from build123d import *

# Parameters (mm, degrees)
BOSS_EXTRUDE1_DEPTH = 6
FILLET1_R           = 3.81
CUT_EXTRUDE1_DEPTH  = 57.584242648


with BuildPart() as part:
    # Sketch1 → Boss-Extrude1 (new body)
    with BuildSketch(Plane.XY):
        Polygon((-12.35, 31.925), (0, 31.925), (0, 37.925), (-6, 37.925), (-6, 34.925), (-9.175, 34.925), (-9.175, 37.925), (-12.35, 37.925), align=None)
        Polygon((19.3548, 12.525), (31.496, 12.525), (31.496, 8.54), (34.496, 8.54), (34.496, 2.54), (31.496, 2.54), (31.496, 0), (25.3548, 0), (25.3548, -6), (19.3548, -6), (19.3548, 0), (0, 0), (0, 44.45), (10.16, 44.45), align=None)
        Polygon((-6, 6.525), (0, 6.525), (0, 12.525), (-12.35, 12.525), (-12.35, 6.525), (-9.175, 6.525), (-9.175, 9.525), (-6, 9.525), align=None)
    extrude(amount=BOSS_EXTRUDE1_DEPTH)

    # Fillet1
    fillet1_edges = [part.edges().sort_by_distance(p)[0] for p in [
        (19.3548, 12.525, 3),
        (0, 0, 3),
    ]]
    fillet(fillet1_edges, radius=FILLET1_R)

    # Sketch3 → Cut-Extrude1 (cut, through all)
    with BuildSketch(Plane.XY.offset(6)):
        Polygon((3.708914399, 34.727201635), (9.47454486, 36.387775447), (7.813971047, 42.153405908), (2.048340586, 40.492832096), align=None)
        Polygon((15.801331085, 14.42072339), (17.461904898, 8.655092929), (11.696274437, 6.994519117), (10.035700624, 12.760149578), align=None)
    extrude(amount=-CUT_EXTRUDE1_DEPTH, mode=Mode.SUBTRACT)


solid = part.part
Part model, mm, in its own coordinate system. A direction names the side the tool comes from. Round coordinates to 2 decimals unless told otherwise and drop trailing zeros. Write each loop counter-clockwise with the first axis right and the second up, starting at its lowest first coordinate (ties: lowest second). Pieces come first, ordered by that corner, then holes. Notation, with made-up numbers: M 77.5,49.5 L 90.5,49.5 A26 ccw 90.5,72.5 Z; hole C -21.75,64 d11. An arc over 180 degrees is marked long. Return JSON: item names as keys, results as strings. Group by question number.
(1) Two-plate mould, pull along Y, no slides. Class faces 1 (the face through (34.496, 6, 3)), 2 (the face through (14.3, 30.07, 2.96)), 3 (the face through (14.619, 7.836, 3.042)): +Y half, -Y half, draft (parallel to the pull), parting line (faces both ways), or undercut.
(2) Which spindle directions (+Z, -Z, +X, -X, +Y, -Y) get a long thin tool onto all of the face, cutting with end or side? Do faces 4 (the face through (-9.175, 8, 3)), 5 (the face through (6.551, 35.546, 3.042)), 6 (the face through (-3, 37.925, 3)), 7 (the face through (0, 22, 3)). Say none if no direction does.
(3) Saw through at D-D on z = 3. Count the separate pieces of the cut face and the enclosed holes in it, then the cut area to 3 significant figures.
(4) Drill centre lines: probe 1 along Y at (x, z) = (-1, 5.75) (3 decimals); probe 2 along X at (y, z) = (-1, 5.5); probe 3 along Y at (x, z) = (4.5, 1.75). Where is each one in solid material? Low to high.
(5) Saw through at A-A on x = -5. Write the cut outline in (y, z) (3 decimals), then the cut area to 3 significant figures.
(6) Pin check, flat tips, straight feed: pin 1 Ø1 at (x, z) = (-11, 4.5) entering from -Y (3 decimals); pin 2 Ø1.6 at (x, z) = (-7, 3) entering from +Y (3 decimals); pin 3 Ø2 at (x, z) = (21.5, 2) entering from +Y. Stop position of each tip, or through.
(7) Saw through at B-B on y = 11. Write the cut outline in (x, z), then the cut area to 3 significant figures.
(8) Saw through at C-C on y = 37. Write the cut outline in (x, z) (3 decimals).
Returned:
{
 "1": {"face 1": "draft", "face 2": "+Y half", "face 3": "undercut"},
 "2": {"face 4": "+Z, -Z, -Y", "face 5": "+Z, -Z", "face 6": "+Z, -Z, -X, +Y", "face 7": "+Z, -Z, -X"},
 "3": {"separate pieces": "1", "enclosed holes": "2", "area": "975 mm²"},
 "4": {"probe 1": "6.525 to 12.525, 31.925 to 37.925", "probe 2": "19.35 to 25.35", "probe 3": "0 to 34.96, 41.2 to 44.45"},
 "5": {"outline": "M 6.525,0 L 12.525,0 L 12.525,6 L 6.525,6 Z; M 31.925,0 L 37.925,0 L 37.925,6 L 31.925,6 Z", "area": "72.0 mm²"},
 "6": {"pin 1": "y = 6.525", "pin 2": "y = 34.925", "pin 3": "y = 12.94"},
 "7": {"outline": "M -12.35,0 L 10.54,0 L 10.54,6 L -12.35,6 Z; M 16.79,0 L 31.5,0 L 31.5,6 L 16.79,6 Z", "area": "226 mm²"},
 "8": {"outline": "M -12.35,0 L -9.175,0 L -9.175,6 L -12.35,6 Z; M -6,0 L 3.054,0 L 3.054,6 L -6,6 Z; M 9.298,0 L 12.306,0 L 12.306,6 L 9.298,6 Z"}
}
